Autodesk Inventor part; units mm, degrees
ref_plane "YZ Plane" through (0, 0, 0) normal (1, 0, 0) x (0, 1, 0)
ref_plane "XZ Plane" through (0, 0, 0) normal (0, 1, 0) x (-1, 0, 0)
ref_plane "XY Plane" through (0, 0, 0) normal (0, 0, 1) x (1, 0, 0)
sketch "スケッチ2" plane through (0, 0, 0) normal (0, 1, 0) x (-1, 0, 0)
  line L0 (0, 0) -> (40, 0)
  line L1 (40, 0) -> (40, -23.7735)
  line L2 (-30, -51.9615) -> (0, 0)
  line L3 (-30, -51.9615) -> (-10, -86.6025)
  line L4 (-10, -86.6025) -> (10.5885, -74.7158)
  line L5 (10.5885, -74.7158) -> (40, -23.7735)
  line L6 (-30, -51.9615) -> (-36.3397, -48.3013) construction
  line L7 (30, 0) -> (30, -18) construction
  line L8 (30, -18) -> (40, -23.7735) construction
  dimension "d0" = 60
  dimension "d1" = 60
  dimension "d2" = 40
  dimension "d3" = 60
  dimension "d4" = 18
  dimension "d5" = 30
  dimension "d6" = 60
extrude "プレート1" add sketch "スケッチ2" along normal blind 1.5
sketch "スケッチ3" plane through (0, 1.5, 0) normal (0, 1, 0) x (1, 0, 0)
  line L0 (-10.5885, 74.7158) -> (-40, 23.7735)
  line L1 (-31.7863, 38) -> (10.9697, 38)
  line L2 (10.9697, 38) -> (19.1969, 33.25)
  line L3 (0, 0) -> (30, 51.9615)
  line L4 (30, 51.9615) -> (0, 0)
  line L5 (0, 0) -> (-40, 0)
  circle A0 centre (0, 50.5) radius 12.5 construction
  circle A1 centre (0, 50.5) radius 1.5
  circle A2 centre (0, 50.5) radius 10.5 construction
  circle A3 centre (5.9346, 70.644) radius 10.5 construction
  circle A4 centre (5.9346, 70.644) radius 11.5 construction
  line L6 (10, 86.6025) -> (30, 51.9615)
  circle A5 centre (5.9346, 70.644) radius 1.5
  line L7 (-30, 0) -> (-30, 18)
  line L8 (-30, 18) -> (-18.453, 38)
  line L9 (-40, 23.7735) -> (-10.5885, 74.7158)
  line L10 (-40, 23.7735) -> (-40, 0)
  line L11 (-40, 23.7735) -> (-30, 18)
  line L12 (-31, 0) -> (-31, 18.5774)
  line L13 (-18.0543, 41) -> (-31, 18.5774)
  line L14 (-18.0543, 41) -> (7.7735, 41)
  line L15 (7.7735, 41) -> (19.6969, 34.116)
  circle A6 centre (0, 50.5) radius 9 construction
  line L16 (-29.7656, 59.5) -> (9, 59.5)
  line L17 (9, 59.5) -> (9, 41.5) construction
  line L18 (9, 41.5) -> (-29.7656, 41.5)
  line L19 (-29.7656, 41.5) -> (-29.7656, 59.5)
  line L20 (-29.7656, 41.5) -> (-19.3733, 59.5)
  line L21 (0, 59.5) -> (0, 41.5)
  dimension "d8" = 38
  dimension "d9" = 9.5
  dimension "d10" = 25
  dimension "d11" = 3
  dimension "d14" = 21
  dimension "d15" = 21
  dimension "d16" = 23
  dimension "d17" = 3
  dimension "d18" = 30
  dimension "d19" = 18
  dimension "d21" = 1
  dimension "d22" = 3
  dimension "d23" = 1
  dimension "d24" = 18
extrude "切り取り1" cut sketch "スケッチ3" against normal blind 1.5 contours L21 A1 | A1 L21 | L13 L14 L15 L3 L2 L1 | L1 L8 L11 L13 | L11 L7 L5 L12 | L1 L2 L3 L5 L7 L8
sketch "スケッチ4" plane through (0, 1.5, 0) normal (0, 1, 0) x (1, 0, 0)
  circle A0 centre (5.1388, 78.0224) radius 1.6
  line L0 (14.0853, 64.5965) -> (11.5853, 60.2663)
  circle A1 centre (13.1994, 68.061) radius 1.6
  circle A2 centre (-36, 15.8638) radius 1.6
  circle A3 centre (20.4199, 44.6683) radius 1.6
  circle A4 centre (24.5152, 51.7615) radius 1.6
  circle A5 centre (-27.8315, 33.15) radius 1.6
  circle A6 centre (-31.9338, 26.0447) radius 1.6
  circle A7 centre (-8.7282, 67.9379) radius 1.6
  circle A8 centre (1.9592, 67.9379) radius 1.6
  line L1 (-31, 18.5774) -> (-31, 0)
  line L2 (-31, 0) -> (-37.5, 0)
  line L3 (-37.5, 0) -> (-37.5, 8)
  line L4 (-37.5, 8) -> (-31, 8)
  line L5 (-31, 8) -> (-31, 0)
  line L6 (-40, 0) -> (-40, 23.7735)
  point P0 (0, 0)
  dimension "d29" = 8
  dimension "d30" = 2.5
extrude "切り取り2" cut sketch "スケッチ4" against normal blind 1.5
fillet "フィレット1" radius 0.5 12 edges at (10, 0.75, -86.6025) (30, 0.75, -51.9615) (-10.5885, 0.75, -74.7158) (-40, 0.75, -23.7735) (-40, 0.75, 0) (-37.5, 0.75, 0) (-37.5, 0.75, -8) (-31, 0.75, -8) (-31, 0.75, -18.5774) (-18.0543, 0.75, -41) (7.7735, 0.75, -41) (19.6969, 0.75, -34.116)
equation "\"d1\" = d0"
equation "\"d12\" = Thickness"
equation "\"d25\" = Thickness"
equation "\"d7\" = Thickness"
properties part number "base_cover" material "アルミニウム 6061"
Can you work these out from the model? Positions are in its coordinate system, mm. A direction names the side the tool comes from. Give positions to 0.01 mm unless a question says otherwise; leave off trailing zeros. Loops run counter-clockwise (first coordinate to the right, second up) from the corner with the lowest first, then second, coordinate; pieces in that order, holes last. Notation, with made-up numbers: (67, -33) - (106, -33) arc R23 cw to (106, -7) - close; hole circle Ø3 at (-19, 62.25). An arc over 180 degrees is marked (long way). One line per item, written item: value.
(1) I need wall thicknesses on line 1 along X through (y, z) = (0.45, -67.5); line 2 along X through (y, z) = (1.45, -13.5); line 3 along X through (y, z) = (0.4, -16.5). Which ranges of each line are inside material? Lowest first, please.
Verdict:
line 1: -14.75 to -10.27, -7.19 to 0.42, 3.5 to 11.7, 14.7 to 21.03
line 2: -40 to -31
line 3: -40 to -37.47, -34.53 to -31
(2) I'm going to push flat-ended pins straight in: pin 1 (3 mm diameter, centred on x = -36, z = -15.86, fed in from -Y); pin 2 (0.8 mm diameter, centred on x = 0, y = 1, fed in from +Z). Where does each tip first touch, or does it pass through?
Verdict:
pin 1: through
pin 2: z = -41
(3) If we section it at A-A, the plane x = 25: List the corners of the cut face in (y, z) for me, plus the area to 3 significant figures.
Verdict:
outline: (0, -60.62) - (1.5, -60.62) - (1.5, -53.29) - (0, -53.29) - close; (0, -50.24) - (1.5, -50.24) - (1.5, -43.3) - (0, -43.3) - close
area: 21.4 mm^2
(4) If we section it at C-C, the plane y = 0.45: State how many separate pieces and enclosed holes the cut face has, plus the area to 3 significant figures.
Verdict:
separate pieces: 1
enclosed holes: 10
area: 2,030 mm^2
(5) If we section it at B-B, the plane z = -33.15: List the corners of the cut face in (x, y) for me.
Verdict:
outline: (-34.59, 0) - (-29.43, 0) - (-29.43, 1.5) - (-34.59, 1.5) - close; (-26.23, 0) - (-22.59, 0) - (-22.59, 1.5) - (-26.23, 1.5) - close
(6) If we section it at D-D, the plane z = -6.5: List the corners of the cut face in (x, y) for me.
Verdict:
outline: (-40, 0) - (-37.5, 0) - (-37.5, 1.5) - (-40, 1.5) - close
(7) On a 3-axis mill with a long thin cutter (end or side, diameter ignored), from which of +Z, -Z, +X, -X, +Y, -Y can I reach the whole of each face in a straight line? I mean faces 4 (the face through (-30.4, 0.8, -26.5)), 5 (the face through (-24.477, 0.76, -29.876)). Say none if no direction works.
Verdict:
face 4: +Y, -Y
face 5: +Z, +Y, -Y
(8) If we mould it in two halves opening along Z, with no side actions, what happens to faces 1 (the face through (-2, 1.5, -49)), 2 (the face through (20.19, 0.74, -68.95)), 3 (the face through (12.991, 0.76, -69.647))? For each: released by +Z, released by -Z, zero draft, split by the parting line, or undercut.
Verdict:
face 1: zero draft
face 2: released by -Z
face 3: undercut
